Read the model definition and answer for the solid it produces. Units are mm, in the model's axes. Face numbers are marked on the shaded views. A direction names the side the tool comes from. Coordinates: 2 decimals unless noted, no trailing zeros. Order: outer loops, then holes, each group sorted by start corner. A loop starts at its lowest first (then second) coordinate and runs counter-clockwise, first axis right, second up. Notation, with made-up numbers: (-12.5, 25.25) -> (4.5, 25.25) arc R18 ccw to (4.5, 43.25) -> close; hole circle Ø3 at (-39, 71.25). An arc over 180 degrees is marked (long way). Use CSV: the item, a comma, the result in double quotes.
```python
from build123d import *

# Parameters (mm, degrees)
F1_DEPTH = 25
F3_R     = 6.5
F4_DEPTH = 87.828853
F5_DEPTH = 30.001
F2_R     = 5.5
F6_DEPTH = 30.001


with BuildPart() as f1:
    # F0 (on Front) → F1 (new body)
    with BuildSketch(Plane.XZ):
        Polygon((0, 30), (0, 0), (39.15558, 0), (39.15558, 17), (74.15558, 17), (74.15558, 0), (113, 0), (113, 30), (87.827853, 30), (87.827853, 64), (68.827853, 64), (68.827853, 30), (43.827853, 30), (43.827853, 64), (24.827853, 64), (24.827853, 30), align=None)
    extrude(amount=F1_DEPTH)

    # F3 (on face) → F4 (cut, through all)
    with BuildSketch(Plane.YZ.offset(87.827853)):
        with Locations((-13.453124, 46)):
            Circle(F3_R)
    extrude(amount=-F4_DEPTH, mode=Mode.SUBTRACT)

    # F2 (on face) → F5 (cut, through all)
    with BuildSketch(Plane.XY.offset(30)):
        Polygon((0, -25), (8.3075, -25), (0, -19.74), align=None)
        Polygon((113, -19.74), (107.418746, -25), (113, -25), align=None)
    extrude(amount=-F5_DEPTH, mode=Mode.SUBTRACT)

    # F2 (on face) → F6 (cut, through all)
    with BuildSketch(Plane.XY.offset(30)):
        Polygon((113, -19.74), (107.418746, -25), (113, -25), align=None)
        Polygon((0, -25), (8.3075, -25), (0, -19.74), align=None)
        with Locations((12.419996, -11.515)):
            Circle(F2_R)
        with Locations((100.413927, -11.515)):
            Circle(F2_R)
    extrude(amount=-F6_DEPTH, mode=Mode.SUBTRACT)


solid = f1.part
```
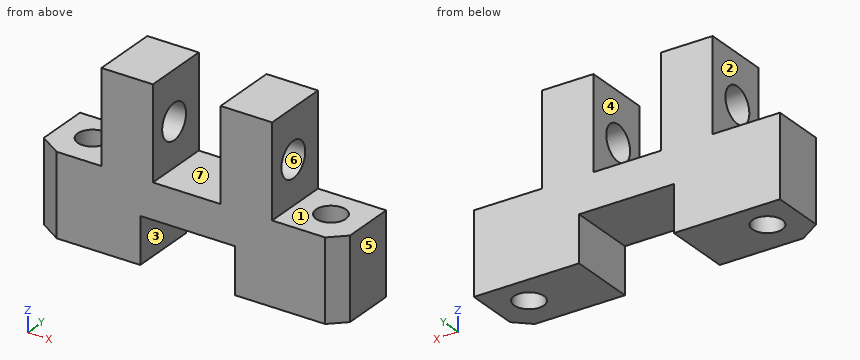
Item 1: The mould has two halves that part along X. Classify the marked faces 5, 6 and 7: +X half, -X half, draft (parallel to the pull), parting line (faces both ways), or undercut.
Return value:
face 5,"+X half"
face 6,"draft"
face 7,"undercut"
Item 2: Find section C-C, the plane y = -15. Give the number of separate pieces and of enclosed holes in the cut face, then the cut area to 3 significant figures.
Return value:
separate pieces,"5"
enclosed holes,"0"
area,"3,100 mm^2"
Item 3: Each of these flat-tipped pins is pushed along its axis until it touches: P1, Ø12, axis at x = 36.5, z = 10.5, coming from the +Y side; P2, Ø4, axis at y = -3, z = 52, coming from the +X side; P3, Ø7.5, axis at y = -14, z = 47, coming from the +X side; P4, Ø12.5, axis at x = 61, y = -17.5, coming from the +Z side. Where does it stop, or does it pass through?
Return value:
P1,"stops at y = 0"
P2,"stops at x = 87.83"
P3,"passes through"
P4,"stops at z = 30"
Item 4: Find section B-B, the plane z = 46. Give the vertices of the cut face in (x, y).
Return value:
outline,"(24.83, -25) -> (43.83, -25) -> (43.83, -19.95) -> (24.83, -19.95) -> close; (24.83, -6.95) -> (43.83, -6.95) -> (43.83, 0) -> (24.83, 0) -> close; (68.83, -25) -> (87.83, -25) -> (87.83, -19.95) -> (68.83, -19.95) -> close; (68.83, -6.95) -> (87.83, -6.95) -> (87.83, 0) -> (68.83, 0) -> close"
Item 5: Straight lines are drawn through the part: line 1 along X through (y, z) = (-17.75, 38.5); line 2 along X through (y, z) = (-12.25, 4.5); line 3 along X through (y, z) = (-11.75, 18). For each, find the intervals that lie inside material, in ascending order.
Return value:
line 1,"x = 24.83 to 43.83, 68.83 to 87.83"
line 2,"x = 0 to 6.97, 17.87 to 39.16, 74.16 to 94.96, 105.86 to 113"
line 3,"x = 0 to 6.93, 17.91 to 94.92, 105.91 to 113"
Item 6: Find section D-D, the plane x = 36.5. Give the vertices of the cut face in (y, z), then the cut area to 3 significant figures.
Return value:
outline,"(-25, 0) -> (0, 0) -> (0, 64) -> (-25, 64) -> close; hole circle Ø13 at (-13.45, 46)"
area,"1,470 mm^2"
Item 7: A tool of negligible diameter and unlimited length cuts with its end or side. For the marked faces 1, 2, 3 and 4, from which of +Z, -Z, +X, -X, +Y, -Y can it reach the whole face along a straight path? Write none if from no direction.
Return value:
face 1,"+Z, +X, +Y, -Y"
face 2,"+Z, -X, +Y, -Y"
face 3,"-Z, +Y, -Y"
face 4,"+Z, +Y, -Y"
Item 8: Find section A-A, the plane z = 33.5. Give the vertices of the cut face in (x, y), then the cut area to 3 significant figures.
Return value:
outline,"(24.83, -25) -> (43.83, -25) -> (43.83, 0) -> (24.83, 0) -> close; (68.83, -25) -> (87.83, -25) -> (87.83, 0) -> (68.83, 0) -> close"
area,"950 mm^2"
